Geometry check sheet. Reference: the model listing, model coordinates, mm. Coordinates: 2 decimals unless noted, no trailing zeros. Loops run counter-clockwise (first coordinate to the right, second up) from the corner with the lowest first, then second, coordinate; pieces in that order, holes last. Notation, with made-up numbers: M -2,-14.5 L 8,-14.5 A23 ccw 8,3.5 Z; hole C 29.5,-32.5 d10. An arc over 180 degrees is marked long. Use CSV: the item, a comma, the result in double quotes.
```python
from build123d import *

# Parameters (mm, degrees)
F1_DEPTH = 2.5
F2_R     = 4
F3_R     = 5
F4_DEPTH = 2.501
F5_R     = 5
F6_DEPTH = 2.501


with BuildPart() as f1:
    # F0 (on Front) → F1 (new body)
    with BuildSketch(Plane.XZ):
        Polygon((77.5, 22.5), (-77.5, 22.5), (-77.5, -22.5), (-22.5, -22.5), (-22.5, -122.5), (22.5, -122.5), (22.5, -22.5), (77.5, -22.5), align=None)
    extrude(amount=F1_DEPTH)

    # F2
    f2_edges = [f1.edges().sort_by_distance(p)[0] for p in [
        (-77.5, -1.25, 22.5),
        (-77.5, -1.25, -22.5),
        (77.5, -1.25, 22.5),
        (77.5, -1.25, -22.5),
        (22.5, -1.25, -122.5),
        (-22.5, -1.25, -122.5),
        (22.5, -1.25, -22.5),
        (-22.5, -1.25, -22.5),
    ]]
    fillet(f2_edges, radius=F2_R)

    # F3 (on face) → F4 (cut, through all)
    with BuildSketch(Plane.XZ.offset(2.5)):
        with Locations((49.5, 0)):
            Circle(F3_R)
        with Locations((-49.5, 0)):
            Circle(F3_R)
        with Locations((0, -92.5)):
            Circle(F3_R)
    extrude(amount=-F4_DEPTH, mode=Mode.SUBTRACT)

    # F5 (on face) → F6 (cut, through all)
    with BuildSketch(Plane.XZ.offset(2.5)):
        with Locations((0, -42.5)):
            Circle(F5_R)
    extrude(amount=-F6_DEPTH, mode=Mode.SUBTRACT)


solid = f1.part
```
1. Release check for a two-part mould opening along X. For faces 1 (the flat face through (-1, 0, -33)), 2 (the cylindrical face through (-76.359, -1.268, -21.297)), 3 (the cylindrical face through (-54.495, -1.268, 0.22)) record: +X half, -X half, draft (parallel to the pull), parting line (faces both ways), or undercut.
The answers:
face 1,"draft"
face 2,"-X half"
face 3,"undercut"
2. Section check C-C, the plane x = 0. Record the cut outline in (y, z).
The answers:
outline,"M -2.5,-122.5 L 0,-122.5 L 0,-97.5 L -2.5,-97.5 Z; M -2.5,-87.5 L 0,-87.5 L 0,-47.5 L -2.5,-47.5 Z; M -2.5,-37.5 L 0,-37.5 L 0,22.5 L -2.5,22.5 Z"
3. Section check B-B, the plane z = -92.5. Record the cut outline in (x, y).
The answers:
outline,"M -22.5,-2.5 L -5,-2.5 L -5,0 L -22.5,0 Z; M 5,-2.5 L 22.5,-2.5 L 22.5,0 L 5,0 Z"
4. Thickness scan on line 1 (Z direction, x = 0.5, y = -2.1); line 2 (X direction, y = -2.1, z = 3); line 3 (Z direction, x = -49.5, y = -0.85). Record the ranges inside material, lowest first. Write a range as [from, to].
The answers:
line 1,"[-122.5, -97.47], [-87.53, -47.47], [-37.53, 22.5]"
line 2,"[-77.5, -53.5], [-45.5, 45.5], [53.5, 77.5]"
line 3,"[-22.5, -5], [5, 22.5]"
5. Section check D-D, the plane y = -1.2. Record the cut outline in (x, z).
The answers:
outline,"M -77.5,-18.5 A4 ccw -73.5,-22.5 L -26.5,-22.5 A4 cw -22.5,-26.5 L -22.5,-118.5 A4 ccw -18.5,-122.5 L 18.5,-122.5 A4 ccw 22.5,-118.5 L 22.5,-26.5 A4 cw 26.5,-22.5 L 73.5,-22.5 A4 ccw 77.5,-18.5 L 77.5,18.5 A4 ccw 73.5,22.5 L -73.5,22.5 A4 ccw -77.5,18.5 Z; hole C -49.5,0 d10; hole C 0,-92.5 d10; hole C 0,-42.5 d10; hole C 49.5,0 d10"
6. Gauge pin test, flat ends, axial feed: P1, Ø0.8, axis at y = -1.5, z = -73.5, coming from the -X side; P2, Ø8, axis at x = 0, z = -92.5, coming from the -Y side; P3, Ø1.2, axis at x = -60.5, y = -1, coming from the -Z side. Record the tip position at first contact, or that the pin passes through.
The answers:
P1,"x = -22.5"
P2,"through"
P3,"z = -22.5"
7. Section check A-A, the plane x = 49.5. Record the cut outline in (y, z).
The answers:
outline,"M -2.5,-22.5 L 0,-22.5 L 0,-5 L -2.5,-5 Z; M -2.5,5 L 0,5 L 0,22.5 L -2.5,22.5 Z"
